Check sheet for the modelled part. Datum: model origin and axes. Units: mm. A direction names the side the tool comes from. Round coordinates to 2 decimals unless told otherwise and drop trailing zeros. Loops run counter-clockwise (first coordinate to the right, second up) from the corner with the lowest first, then second, coordinate; pieces in that order, holes last. Notation, with made-up numbers: (22, -15) -> (69, -15) arc R11 ccw to (69, -3) -> close; hole circle Ø8 at (20.5, 5.25). An arc over 180 degrees is marked (long way). One line per question, with ' | ' between items.
```python
from build123d import *

# Parameters (mm, degrees)
BOSS_EXTRUDE1_DEPTH     = 12.065
CUT_EXTRUDE1_DEPTH      = 13.065
CUT_EXTRUDE1_DEPTH_BACK = 13.065
SKETCH3_R               = 2.54
SKETCH3_R_2             = 1.477926828
BOSS_EXTRUDE2_DEPTH     = 4.1275


with BuildPart() as part:
    # Sketch1 → Boss-Extrude1 (new body, symmetric)
    with BuildSketch(Plane.XY):
        with BuildLine():
            ThreePointArc((-3.256590116, -1.261814988), (-2.469570433, -2.469570433), (-1.261814988, -3.256590116))
            ThreePointArc((-1.261814988, -3.256590116), (0, -2.921), (1.261814988, -3.256590116))
            ThreePointArc((1.261814988, -3.256590116), (2.469570433, -2.469570433), (3.256590116, -1.261814988))
            ThreePointArc((3.256590116, -1.261814988), (2.921, 0), (3.256590116, 1.261814988))
            ThreePointArc((3.256590116, 1.261814988), (2.469570433, 2.469570433), (1.261814988, 3.256590116))
            ThreePointArc((1.261814988, 3.256590116), (0, 2.921), (-1.261814988, 3.256590116))
            ThreePointArc((-1.261814988, 3.256590116), (-2.469570433, 2.469570433), (-3.256590116, 1.261814988))
            ThreePointArc((-3.256590116, 1.261814988), (-2.921, 0), (-3.256590116, -1.261814988))
        make_face()
    extrude(amount=BOSS_EXTRUDE1_DEPTH, both=True)

    # Sketch2 → Cut-Extrude1 (cut, two sides)
    with BuildSketch(Plane.XY) as cut_extrude1_sk:
        with BuildLine():
            Line((-0.898025612, 2.375952441), (0, 1.477926828))
            Line((0, 1.477926828), (0.898025612, 2.375952441))
            ThreePointArc((0.898025612, 2.375952441), (1.796051224, 1.796051224), (2.375952441, 0.898025612))
            Line((2.375952441, 0.898025612), (1.477926828, 0))
            Line((1.477926828, 0), (2.375952441, -0.898025612))
            ThreePointArc((2.375952441, -0.898025612), (1.796051224, -1.796051224), (0.898025612, -2.375952441))
            Line((0.898025612, -2.375952441), (0, -1.477926828))
            Line((0, -1.477926828), (-0.898025612, -2.375952441))
            ThreePointArc((-0.898025612, -2.375952441), (-1.796051224, -1.796051224), (-2.375952441, -0.898025612))
            Line((-2.375952441, -0.898025612), (-1.477926828, 0))
            Line((-1.477926828, 0), (-2.375952441, 0.898025612))
            ThreePointArc((-2.375952441, 0.898025612), (-1.796051224, 1.796051224), (-0.898025612, 2.375952441))
        make_face()
    extrude(amount=CUT_EXTRUDE1_DEPTH, mode=Mode.SUBTRACT)
    extrude(cut_extrude1_sk.sketch, amount=-CUT_EXTRUDE1_DEPTH_BACK, mode=Mode.SUBTRACT)

    # Sketch3 → Boss-Extrude2 (add, symmetric)
    with BuildSketch(Plane.XY):
        Circle(SKETCH3_R)
        Circle(SKETCH3_R_2, mode=Mode.SUBTRACT)
    extrude(amount=BOSS_EXTRUDE2_DEPTH, both=True)


solid = part.part
```
(1) Scan lines: probe 1 along X at (y, z) = (-2, -8.5); probe 2 along Y at (x, z) = (0, 1.5); probe 3 along X at (y, z) = (1.75, 10.5). Record each from-to range of solid material in increasing order.
Answer:
probe 1: x = -2.86 to -1.57, -0.52 to 0.52, 1.57 to 2.86 | probe 2: y = -2.92 to -1.48, 1.48 to 2.92 | probe 3: x = -3.02 to -1.84, -0.27 to 0.27, 1.84 to 3.02
(2) Sectioned sample at A-A, the plane z = 0.75. Record the cut outline in (x, y) (1 decimal), and give its area (3 significant figures).
Answer:
outline: (-3.3, -1.3) arc R3.5 ccw to (-1.3, -3.3) arc R2.5 cw to (1.3, -3.3) arc R3.5 ccw to (3.3, -1.3) arc R2.5 cw to (3.3, 1.3) arc R3.5 ccw to (1.3, 3.3) arc R2.5 cw to (-1.3, 3.3) arc R3.5 ccw to (-3.3, 1.3) arc R2.5 cw to start; hole circle Ø3 at (0, 0) | area: 27.6 mm2
(3) Set-up check for faces 1 (the face through (-1.933, -0.455, -8.041)), 2 (the face through (1.4, 1.5, 4.128)), 3 (the face through (2.46, -2.48, 0.17)): record each of +Z, -Z, +X, -X, +Y, -Y from which the full face is reachable in a straight line by a thin tool's end or side.
Answer:
face 1: -Z | face 2: +Z | face 3: +Z, -Z, +X, -Y
(4) Sectioned sample at B-B, the plane x = 0.5. Record the cut outline in (y, z) (1 decimal).
Answer:
outline: (-3, -12.1) -> (-2, -12.1) -> (-2, -4.1) -> (-1.4, -4.1) -> (-1.4, 4.1) -> (-2, 4.1) -> (-2, 12.1) -> (-3, 12.1) -> close; (1.4, -4.1) -> (2, -4.1) -> (2, -12.1) -> (3, -12.1) -> (3, 12.1) -> (2, 12.1) -> (2, 4.1) -> (1.4, 4.1) -> close
(5) Mould release check, pull along X, two halves, no side actions. Record for faces 4 (the face through (-2.46, 2.48, 0.17)), 5 (the face through (-0.02, -2.92, 0.17)), 6 (the face through (2.92, -0.02, 0.17)): +X half, -X half, draft (parallel to the pull), parting line (faces both ways), or undercut.
Answer:
face 4: -X half | face 5: undercut | face 6: +X half
(6) Sectioned sample at D-D, the plane y = -2. Record the cut outline in (x, z) (1 decimal).
Answer:
outline: (-2.9, -12.1) -> (-1.6, -12.1) -> (-1.6, -4.1) -> (-0.5, -4.1) -> (-0.5, -12.1) -> (0.5, -12.1) -> (0.5, -4.1) -> (1.6, -4.1) -> (1.6, -12.1) -> (2.9, -12.1) -> (2.9, 12.1) -> (1.6, 12.1) -> (1.6, 4.1) -> (0.5, 4.1) -> (0.5, 12.1) -> (-0.5, 12.1) -> (-0.5, 4.1) -> (-1.6, 4.1) -> (-1.6, 12.1) -> (-2.9, 12.1) -> close
(7) Go/stop test with flat-tipped pins: pin 1 (1 mm diameter, centred on x = 2, z = 1.5, fed in from -Y); pin 2 (1.2 mm diameter, centred on x = -0.5, y = -1, fed in from +Z); pin 3 (0.7 mm diameter, centred on x = 1, y = -1, fed in from -Z). Record where each tip stops, or that it passes through.
Answer:
pin 1: stops at y = -3.15 | pin 2: stops at z = 4.13 | pin 3: stops at z = -4.13
(8) Sectioned sample at C-C, the plane z = -8.75. Record the cut outline in (x, y) (1 decimal), and give its area (3 significant figures).
Answer:
outline: (-3.3, -1.3) arc R3.5 ccw to (-1.3, -3.3) arc R2.5 cw to (1.3, -3.3) arc R3.5 ccw to (3.3, -1.3) arc R2.5 cw to (3.3, 1.3) arc R3.5 ccw to (1.3, 3.3) arc R2.5 cw to (-1.3, 3.3) arc R3.5 ccw to (-3.3, 1.3) arc R2.5 cw to start; hole (-2.4, -0.9) arc R2.5 ccw to (-0.9, -2.4) -> (0, -1.5) -> (0.9, -2.4) arc R2.5 ccw to (2.4, -0.9) -> (1.5, 0) -> (2.4, 0.9) arc R2.5 ccw to (0.9, 2.4) -> (0, 1.5) -> (-0.9, 2.4) arc R2.5 ccw to (-2.4, 0.9) -> (-1.5, 0) -> close | area: 18.2 mm2
